Autodesk Inventor part; units mm, degrees
ref_plane "YZ Plane" through (0, 0, 0) normal (1, 0, 0) x (0, 1, 0)
ref_plane "XZ Plane" through (0, 0, 0) normal (0, 1, 0) x (-1, 0, 0)
ref_plane "XY Plane" through (0, 0, 0) normal (0, 0, 1) x (1, 0, 0)
sketch "Esboço1" plane through (0, 0, 0) normal (0, 0, 1) x (1, 0, 0)
  line L0 (-12.5, 10) -> (12.5, 10)
  line L1 (12.5, 10) -> (12.5, -10)
  line L2 (12.5, -10) -> (-12.5, -10)
  line L3 (-12.5, -10) -> (-12.5, 10)
  line L4 (-12.5, 10) -> (12.5, -10) construction
  line L5 (12.5, 10) -> (-12.5, -10) construction
  point P0 (0, 0)
  dimension "d1" = 20
  dimension "d2" = 25
extrude "Extrusão1" add sketch "Esboço1" along normal mid plane 7
fillet "Arredondamento1" radius 1 4 edges at (12.5, -10, 0) (-12.5, -10, 0) (12.5, 10, 0) (-12.5, 10, 0)
fillet "Arredondamento2" radius 1 16 edges at (12.2071, 9.7071, 3.5) (0, 10, 3.5) (-12.2071, 9.7071, 3.5) (-12.5, 0, 3.5) (-12.2071, -9.7071, 3.5) (0, -10, 3.5) (12.2071, -9.7071, 3.5) (12.5, 0, 3.5) (-12.2071, 9.7071, -3.5) (0, 10, -3.5) (12.2071, 9.7071, -3.5) (12.5, 0, -3.5) (12.2071, -9.7071, -3.5) (0, -10, -3.5) (-12.2071, -9.7071, -3.5) (-12.5, 0, -3.5)
sketch "Esboço6" plane through (-11.5, 10, -2.5) normal (0, 1, 0) x (1, 0, 0)
  circle A0 centre (2, -2.1) radius 0.6
  circle A1 centre (2, -3.5) radius 0.6
  line L0 (0, 0) -> (23, 0)
  line L1 (-1, -5) -> (0, -5)
  line L2 (0, 0) -> (0, -5) construction
  line L3 (23, -5) -> (0, -5)
  point P0 (11.5, -2.5)
  dimension "d24" = 1.2
  dimension "d25" = 2
  dimension "d26" = 2
  dimension "d27" = 1.5
  dimension "d28" = 1.5
  dimension "d29" = 0.2
extrude "Extrusão5" add sketch "Esboço6" along normal blind 5
properties part number "Bateria"
Build history of the part. All positions in model axes, mm. Round coordinates to 2 decimals unless told otherwise and drop trailing zeros. Order: outer loops, then holes, each group sorted by start corner. A loop starts at its lowest first (then second) coordinate and runs counter-clockwise, first axis right, second up. Notation, with made-up numbers: M 37,53.25 L 54,53.25 A20 cw 54,77.25 Z; hole C 74,-17.75 d4. An arc over 180 degrees is marked long. Use CSV: the item, a comma, the result in double quotes. Start each with the question number.
(1) Mould opens along Z. For faces 1 (the face through (0, 0, 3.5)), 2 (the face through (-10.1, 12.5, -0.4)), 3 (the face through (-9.5, 15, 1)) say: +Z half, -Z half, draft (parallel to the pull), parting line (faces both ways), or undercut.
(2) Cut at B-B on x = -9.5. List the corners of the cut face in (y, z).
(3) Drill centre lines: probe 1 along Y at (x, z) = (-3, -0.75); probe 2 along Y at (x, z) = (3, 3); probe 3 along X at (y, z) = (9.5, 2.5). Where is each one in solid material? Low to high.
(4) Flat gauge pins, fed straight in: P1, Ø1.5, axis at x = -6, y = 12.5, coming from the -Z side; P2, Ø2.5, axis at x = 3.5, z = -0.5, coming from the +Y side; P3, Ø1.5, axis at y = 11, z = -1, coming from the +X side. Where does each tip first touch, or does it go through?
(5) Cut at C-C on y = 13.75. List the corners of the cut face in (x, z), then the cut area to 3 significant figures.
(6) Cut at D-D on x = -4.25. List the corners of the cut face in (y, z).
(7) Cut at A-A on z = 2. List the corners of the cut face in (x, y).
Findings:
1,face 1,"+Z half"
1,face 2,"undercut"
1,face 3,"draft"
2,outline,"M -10,-2.5 A1 ccw -9,-3.5 L 9,-3.5 A1 ccw 10,-2.5 L 10,-1 L 15,-1 L 15,0.2 L 10,0.2 L 10,0.4 L 15,0.4 L 15,1.6 L 10,1.6 L 10,2.5 A1 ccw 9,3.5 L -9,3.5 A1 ccw -10,2.5 Z"
3,probe 1,"y = -10 to 10"
3,probe 2,"y = -9.87 to 9.87"
3,probe 3,"x = -12.37 to 12.37"
4,P1,"passes through"
4,P2,"stops at y = 10"
4,P3,"stops at x = -8.9"
5,outline,"C -9.5,-0.4 d1.2; C -9.5,1 d1.2"
5,area,"2.26 mm^2"
6,outline,"M -10,-2.5 A1 ccw -9,-3.5 L 9,-3.5 A1 ccw 10,-2.5 L 10,2.5 A1 ccw 9,3.5 L -9,3.5 A1 ccw -10,2.5 Z"
7,outline,"M -12.5,-9 A1 ccw -11.5,-10 L 11.5,-10 A1 ccw 12.5,-9 L 12.5,9 A1 ccw 11.5,10 L -11.5,10 A1 ccw -12.5,9 Z"
